The figure shows three views and two pictorial views of one solid part (mm, origin at its lowest corner). Answer the questions. Coordinates: 2 decimals unless noted, no trailing zeros. Loops run counter-clockwise (first coordinate to the right, second up) from the corner with the lowest first, then second, coordinate; pieces in that order, holes last.
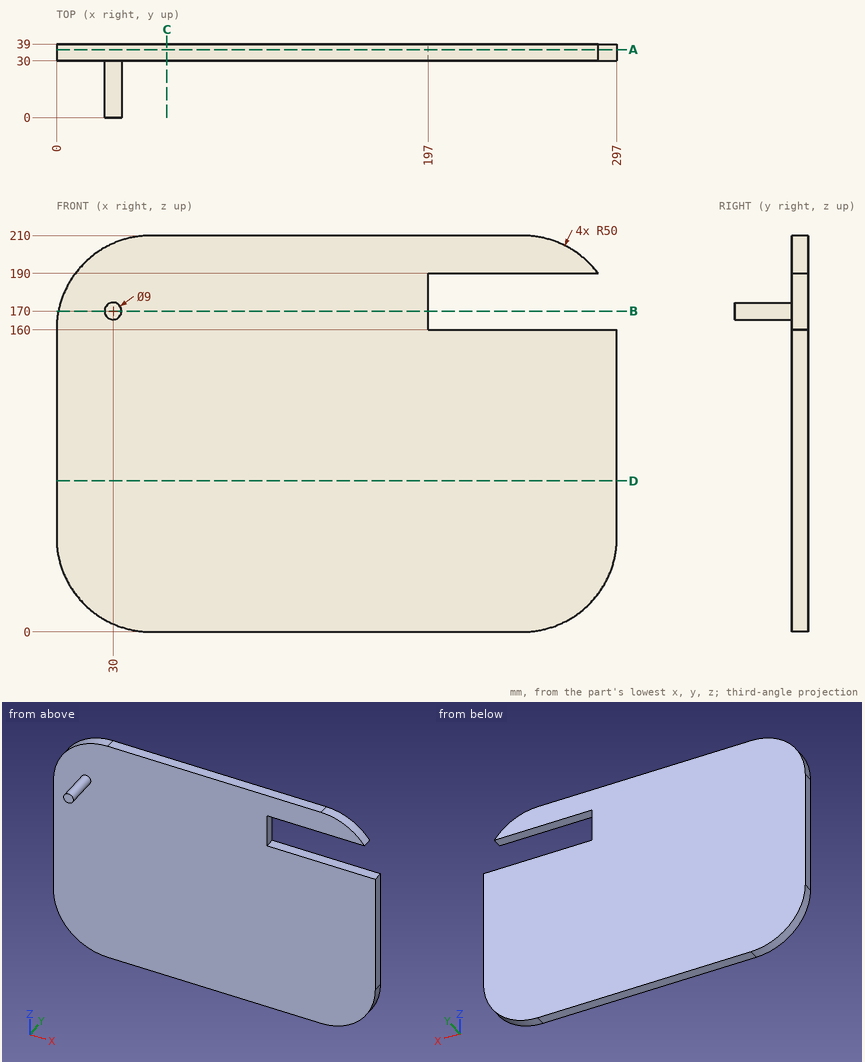
Q1. A cutting plane is placed at C-C (x = 58.5). Give the vertices of the cut face in (y, z).
Findings below:
outline: (30, 0) - (39, 0) - (39, 210) - (30, 210) - close
Q2. A cutting plane is placed at B-B (z = 170). Give the vertices of the cut face in (x, y).
Findings below:
outline: (1.01, 30) - (25.5, 30) - (25.5, 0) - (34.5, 0) - (34.5, 30) - (197, 30) - (197, 39) - (1.01, 39) - close
Q3. A cutting plane is placed at D-D (z = 80). Give the vertices of the cut face in (x, y), then the cut area to 3 significant figures.
Findings below:
outline: (0, 30) - (297, 30) - (297, 39) - (0, 39) - close
area: 2,670 mm2
Q4. A straight line is drawn through the part: probe 1 along Y at (x, z) = (149.5, 36.5). Find the intervals that lie inside material, in ascending order.
Findings below:
probe 1: y = 30 to 39
Q5. A cutting plane is placed at A-A (y = 36). Give the vertices of the cut face in (x, z).
Findings below:
outline: (0, 50) arc R50 ccw to (50, 0) - (247, 0) arc R50 ccw to (297, 50) - (297, 160) - (197, 160) - (197, 190) - (287, 190) arc R50 ccw to (247, 210) - (50, 210) arc R50 ccw to (0, 160) - close
Q6. Flat-ended cylindrical pins translate along their axes: pin 1 Ø7 at (x, y) = (252, 36.5) entering from -Z; pin 2 Ø10 at (y, z) = (33.5, 167.5) entering from +X; pin 3 Ø12 at (x, z) = (240, 133.5) entering from -Y. Find the tip coordinate at first contact, or state that the pin passes through.
Findings below:
pin 1: stops at z = 0.02
pin 2: stops at x = 197
pin 3: stops at y = 30
